```python
from build123d import *

# Parameters (mm, degrees)
SKETCH2_W             = 38.1
SKETCH2_H             = 38.1
SKETCH2_R             = 9.525
BOSS_EXTRUDE1_DEPTH   = 9.525
M4X0_7_TAPPED_HOLE1_D = 3.3


with BuildPart() as part:
    # Sketch2 → Boss-Extrude1 (new body)
    with BuildSketch(Plane(origin=(0, 0, 0), x_dir=(0, 0, -1), z_dir=(1, 0, 0))):
        with Locations((19.05, 19.05)):
            Rectangle(SKETCH2_W, SKETCH2_H)
        with Locations((19.05, 19.05)):
            Circle(SKETCH2_R, mode=Mode.SUBTRACT)
    extrude(amount=BOSS_EXTRUDE1_DEPTH)

    # M4x0.7 Tapped Hole1 (through all)
    with Locations(Plane(origin=(0, 0, -38.1), x_dir=(-1, 0, 0), z_dir=(0, 0, -1))):
        with Locations((-4.7625, 33.3375), (-4.7625, 4.7625)):
            Hole(M4X0_7_TAPPED_HOLE1_D / 2)


solid = part.part
```
Geometry check sheet. Reference: the model listing, model coordinates, mm. Round coordinates to 2 decimals unless told otherwise and drop trailing zeros. Loops run counter-clockwise (first coordinate to the right, second up) from the corner with the lowest first, then second, coordinate; pieces in that order, holes last. Notation, with made-up numbers: (-30.75, 85.5) - (-5.75, 85.5) arc R36 cw to (-5.75, 123.5) - close; hole circle Ø8 at (28.25, -17.5). An arc over 180 degrees is marked (long way). Write each question's results on one line, items separated by ' | '. Start each with the question number.
Q1. Cross-section at A-A on y = 19.05. Enter the section's corners in (x, z) (3 decimals).
Q2. Cross-section at B-B on x = 5.5. State how many separate pieces and enclosed holes the cut face has, and give its area (3 significant figures).
Q3. Release check for a two-part mould opening along Y. For faces 1 (the flat face through (5, 0, -19)), 2 (the flat face through (9.525, 28, -15)), 3 (the cylindrical face through (4.55, 6.4, -18.78)) record: +Y half, -Y half, draft (parallel to the pull), parting line (faces both ways), or undercut.
Q4. Thickness scan on line 1 (Y direction, x = 3.75, z = -8.5); line 2 (Y direction, x = 4.5, z = -16.5); line 3 (Y direction, x = 6.25, z = -34). Record the ranges inside material, lowest first. Write a range as [from, to].
Answers below:
1) outline: (0, -38.1) - (9.525, -38.1) - (9.525, -28.575) - (0, -28.575) - close; (0, -9.525) - (9.525, -9.525) - (9.525, 0) - (0, 0) - close
2) separate pieces: 3 | enclosed holes: 1 | area: 942 mm²
3) face 1: -Y half | face 2: draft | face 3: undercut
4) line 1: y = [0, 3.46], [6.07, 32.03], [34.64, 38.1] | line 2: y = [0, 3.13], [6.39, 9.87], [28.23, 31.71], [34.97, 38.1] | line 3: y = [0, 4.05], [5.48, 32.62], [34.05, 38.1]
